```python
from build123d import *

# Parameters (mm, degrees)
SKETCH_1_W             = 120
SKETCH_1_H             = 45
EXTRUDE_1_DEPTH        = 30
CUT_EXTRUDE_1_REACH    = 72.755
SKETCH_2_R             = 9.5
SKETCH_2_R_2           = 10.75
HOLE_WIZARD_M4_1_D     = 3.3
HOLE_WIZARD_M4_1_DEPTH = 10.1
HOLE_WIZARD_M4_1_TIP   = 0.991420021
HOLE_WIZARD_M4_2_D     = 3.3
HOLE_WIZARD_M4_2_DEPTH = 10.1
HOLE_WIZARD_M4_2_TIP   = 0.991420021
HOLE_WIZARD_M3_1_D     = 2.5
HOLE_WIZARD_M3_1_DEPTH = 7.5
HOLE_WIZARD_M3_1_TIP   = 0.751075774


with BuildPart() as part:
    # 草图1 → 凸台-拉伸1 (new body)
    with BuildSketch(Plane.XY):
        Rectangle(SKETCH_1_W, SKETCH_1_H)
    extrude(amount=EXTRUDE_1_DEPTH)

    # 草图2 → 切除-拉伸1 (cut, up to next)
    with BuildSketch(Plane.XY.offset(30), mode=Mode.PRIVATE) as cut_extrude_1_sk1:
        with Locations((-35, 0)):
            Circle(SKETCH_2_R)
    cut_extrude_1_tool1 = extrude(cut_extrude_1_sk1.sketch, amount=-CUT_EXTRUDE_1_REACH, mode=Mode.PRIVATE) & part.part
    # 草图2 → 切除-拉伸1 (cut, up to next)
    with BuildSketch(Plane.XY.offset(30), mode=Mode.PRIVATE) as cut_extrude_1_sk2:
        with Locations((35, 0)):
            Circle(SKETCH_2_R)
    cut_extrude_1_tool2 = extrude(cut_extrude_1_sk2.sketch, amount=-CUT_EXTRUDE_1_REACH, mode=Mode.PRIVATE) & part.part
    # 草图2 → 切除-拉伸1 (cut, up to next)
    with BuildSketch(Plane.XY.offset(30), mode=Mode.PRIVATE) as cut_extrude_1_sk3:
        Circle(SKETCH_2_R_2)
    cut_extrude_1_tool3 = extrude(cut_extrude_1_sk3.sketch, amount=-CUT_EXTRUDE_1_REACH, mode=Mode.PRIVATE) & part.part
    add(cut_extrude_1_tool1.solids().sort_by_distance((-35, 0, 30))[0], mode=Mode.SUBTRACT)
    add(cut_extrude_1_tool2.solids().sort_by_distance((35, 0, 30))[0], mode=Mode.SUBTRACT)
    add(cut_extrude_1_tool3.solids().sort_by_distance((0, 0, 30))[0], mode=Mode.SUBTRACT)

    # M4 螺纹孔1
    with Locations(Plane.XY.offset(30)):
        with Locations((23.7, 11.3), (-35, 0), (-23.7, 11.3), (-46.3, -11.3), (-46.3, 11.3), (-23.7, -11.3), (46.3, 11.3), (46.3, -11.3), (23.7, -11.3)):
            Hole(HOLE_WIZARD_M4_1_D / 2, depth=HOLE_WIZARD_M4_1_DEPTH)
            with Locations((0, 0, -(HOLE_WIZARD_M4_1_DEPTH + HOLE_WIZARD_M4_1_TIP / 2))):  # 118° drill point
                Cone(0, HOLE_WIZARD_M4_1_D / 2, HOLE_WIZARD_M4_1_TIP, mode=Mode.SUBTRACT)

    # M4 螺纹孔2
    with Locations(Plane(origin=(0, 0, 0), x_dir=(-1, 0, 0), z_dir=(0, 0, -1))):
        with Locations((11.313708499, 11.313708499), (-11.313708499, -11.313708499), (-11.313708499, 11.313708499), (11.313708499, -11.313708499)):
            Hole(HOLE_WIZARD_M4_2_D / 2, depth=HOLE_WIZARD_M4_2_DEPTH)
            with Locations((0, 0, -(HOLE_WIZARD_M4_2_DEPTH + HOLE_WIZARD_M4_2_TIP / 2))):  # 118° drill point
                Cone(0, HOLE_WIZARD_M4_2_D / 2, HOLE_WIZARD_M4_2_TIP, mode=Mode.SUBTRACT)

    # M3 螺纹孔1
    with Locations(Plane(origin=(0, -22.5, 0), x_dir=(-1, 0, 0), z_dir=(0, -1, 0))):
        with Locations((-40.606601718, -4.393398282), (-19.393398282, -4.393398282), (-19.393398282, -25.606601718), (-40.606601718, -25.606601718), (19.393398282, -4.393398282), (40.606601718, -4.393398282), (19.393398282, -25.606601718), (40.606601718, -25.606601718)):
            Hole(HOLE_WIZARD_M3_1_D / 2, depth=HOLE_WIZARD_M3_1_DEPTH)
            with Locations((0, 0, -(HOLE_WIZARD_M3_1_DEPTH + HOLE_WIZARD_M3_1_TIP / 2))):  # 118° drill point
                Cone(0, HOLE_WIZARD_M3_1_D / 2, HOLE_WIZARD_M3_1_TIP, mode=Mode.SUBTRACT)


solid = part.part
```
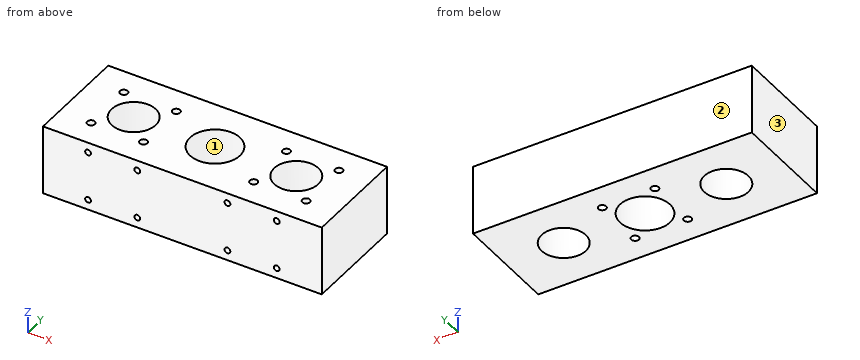
Build history of the part. All positions in model axes, mm. Face numbers are marked on the shaded views. Round coordinates to 2 decimals unless told otherwise and drop trailing zeros. Loops run counter-clockwise (first coordinate to the right, second up) from the corner with the lowest first, then second, coordinate; pieces in that order, holes last.
Item 1: Saw through at D-D (y = 3.5). List the corners of the cut face in (x, z), then the cut area to 3 significant figures.
Item 2: Drill centre lines: line 1 along Y through (x, z) = (-35, 11.5); line 2 along X through (y, z) = (2, 23.25); line 3 along X through (y, z) = (4, 25.5). Where is each one in solid material? Low to high.
Item 3: Saw through at A-A (x = -35). List the corners of the cut face in (y, z).
Item 4: Saw through at B-B (z = 13.25). List the corners of the cut face in (x, y).
Item 5: Pin check, flat tips, straight feed: P1, Ø3, axis at x = -23.7, y = -11.3, coming from the +Z side; P2, Ø17, axis at x = 0, y = 0, coming from the +Z side. Stop position of each tip, or through.
Item 6: Saw through at C-C (z = 22). State how many separate pieces and enclosed holes the cut face has, then the cut area to 3 significant figures.
Item 7: Two-plate mould, pull along Y, no slides. Class the marked faces 1, 2 and 3: released by +Y, released by -Y, zero draft, split by the parting line, or undercut.
Worked answers:
1. outline: (-60, 0) - (-43.83, 0) - (-43.83, 30) - (-60, 30) - close; (-26.17, 0) - (-10.16, 0) - (-10.16, 30) - (-26.17, 30) - close; (10.16, 0) - (26.17, 0) - (26.17, 30) - (10.16, 30) - close; (43.83, 0) - (60, 0) - (60, 30) - (43.83, 30) - close
1. area: 1,930 mm2
2. line 1: y = -22.5 to -9.5, 9.5 to 22.5
2. line 2: x = -60 to -44.29, -25.71 to -10.56, 10.56 to 25.71, 44.29 to 60
2. line 3: x = -60 to -43.62, -26.38 to -9.98, 9.98 to 26.38, 43.62 to 60
3. outline: (-22.5, 0) - (-9.5, 0) - (-9.5, 30) - (-22.5, 30) - close; (9.5, 0) - (22.5, 0) - (22.5, 30) - (9.5, 30) - close
4. outline: (-60, -22.5) - (60, -22.5) - (60, 22.5) - (-60, 22.5) - close; hole circle Ø19 at (-35, 0); hole circle Ø21.5 at (0, 0); hole circle Ø19 at (35, 0)
5. P1: stops at z = 19.81
5. P2: passes through
6. separate pieces: 1
6. enclosed holes: 11
6. area: 4,400 mm2
7. face 1: undercut
7. face 2: released by +Y
7. face 3: zero draft
